Autodesk Fusion 360 part; units mm, degrees
sketch "Sketch1" plane through (0, 0, 0) normal (1, 0, 0) x (0, 1, 0)
  line L0 (15.2, 10) -> (-15.2, 10)
  line L1 (-15.2, 10) -> (-15.2, -10)
  line L2 (-15.2, -10) -> (15.2, -10)
  line L3 (15.2, -10) -> (15.2, 10)
  line L4 (15.2, 10) -> (-15.2, -10) construction
  line L5 (-15.2, 10) -> (15.2, -10) construction
  line L6 (0, 10) -> (0, -10)
  line L7 (15.2, 10) -> (15.2, 8.5)
  line L8 (15.2, 8.5) -> (13.7, 8.5)
  line L9 (13.7, 8.5) -> (13.7, 6.5)
  line L10 (13.7, 6.5) -> (15.2, 6.5)
  line L11 (15.2, -10) -> (15.2, -8.5)
  line L12 (15.2, -8.5) -> (13.7, -8.5)
  line L13 (13.7, -8.5) -> (13.7, -6.5)
  line L14 (13.7, -6.5) -> (15.2, -6.5)
  line L15 (15.2, -6.5) -> (15.2, -5)
  line L16 (15.2, -5) -> (13.2, -5)
  line L17 (15.2, 6.5) -> (15.2, 5)
  line L18 (15.2, 5) -> (13.2, 5)
  line L19 (13.2, 5) -> (13.2, -5)
  dimension "d1" = 30.4
  dimension "d2" = 20
  dimension "d3" = 1.5
  dimension "d4" = 1.5
  dimension "d5" = 2
  dimension "d6" = 1.5
  dimension "d7" = 1.5
  dimension "d8" = 2
  dimension "d9" = 1.5
  dimension "d10" = 2
  dimension "d11" = 2
revolve "Revolve1" add sketch "Sketch1" angle 360 about axis through (0, 0, 10) along (0, 0, -1) contours L0 L2 L3 L6 L7 L8 L9 L10 L11 L12 L13 L14 L15 L16 L17 L18 L19
sketch "Sketch2" plane through (0, 0, 10) normal (0, 0, 1) x (-1, 0, 0)
  circle A0 centre (0, 0) radius 15.2
  line L0 (5.588, -5.588) -> (-5.588, -5.588)
  line L1 (-5.588, -5.588) -> (-5.588, 5.588)
  line L2 (-5.588, 5.588) -> (5.588, 5.588)
  line L3 (5.588, 5.588) -> (5.588, -5.588)
  line L4 (5.588, -5.588) -> (-5.588, 5.588) construction
  line L5 (-5.588, -5.588) -> (5.588, 5.588) construction
  circle A1 centre (5.588, -5.588) radius 1.5875
  dimension "d13" = 11.176
  dimension "d14" = 11.176
  dimension "d15" = 3.175
extrude "Extrude1" cut sketch "Sketch2" against normal blind 25 contours L0 L3 A1 | L0 L3 A1
pattern_circular "C-Pattern1" count 4 over 360 about axis through (0, 0, 1.75) along (0, 0, 1) of "Extrude1"
chamfer "Chamfer1" distance 1.5 angle 45 1 edges at (-12.7729, 4.9541, -8.5)
chamfer "Chamfer2" distance 2 angle 45 1 edges at (-12.3067, 4.7733, -5)
chamfer "Chamfer3" distance 1.5 angle 45 1 edges at (-12.7729, 4.9541, 6.5)
sketch "Sketch3" plane through (0, 0, -10) normal (0, 0, -1) x (1, 0, 0)
  circle A0 centre (5.588, -5.588) radius 1.5875
  circle A1 centre (5.588, 5.588) radius 1.5875
  circle A2 centre (-5.588, 5.588) radius 1.5875
  circle A3 centre (-5.588, -5.588) radius 1.5875
  circle A4 centre (0, 0) radius 15.2
  circle A5 centre (-5.588, 5.588) radius 2.5
  circle A6 centre (-5.588, -5.588) radius 2.5
  circle A7 centre (5.588, -5.588) radius 2.5
  circle A8 centre (5.588, 5.588) radius 2.5
  dimension "d23" = 5
  dimension "d24" = 5
  dimension "d25" = 5
  dimension "d26" = 5
extrude "Extrude2" cut sketch "Sketch3" against normal blind 15 contours A5 | A6 | A7 | A8
sketch "Sketch4" plane through (0, 0, 10) normal (0, 0, 1) x (-1, 0, 0)
  circle A0 centre (-5.588, -5.588) radius 1.5875
  circle A1 centre (-5.588, 5.588) radius 1.5875
  circle A2 centre (5.588, 5.588) radius 1.5875
  circle A3 centre (5.588, -5.588) radius 1.5875
  circle A4 centre (0, 0) radius 15.2
  circle A5 centre (0, 0) radius 4.7625
  dimension "d29" = 9.525
extrude "Extrude3" cut sketch "Sketch4" against normal blind 26 contours A5
equation "d13 = 0.315 in + 0.125 in"
equation "d14 = 0.315 in + 0.125 in"
Verification items for the finished model (mm, model axes). A direction names the side the tool comes from. Give positions to 0.01 mm unless a question says otherwise; leave off trailing zeros. Write each loop counter-clockwise with the first axis right and the second up, starting at its lowest first coordinate (ties: lowest second). Pieces come first, ordered by that corner, then holes.
(1) Mould release check, pull along Y, two halves, no side actions. Record for faces 1 (the face through (3.78, 2.9, 0.14)), 2 (the face through (3.75, -7.28, -2.61)), 3 (the face through (4, 3, 10)), 4 (the face through (-0.668, -15.185, -5.74)): +Y half, -Y half, draft (parallel to the pull), parting line (faces both ways), or undercut.
(2) Gauge pin test, flat ends, axial feed: pin 1 (3 mm diameter, centred on x = 5.588, y = -5.588, fed in from +Z); pin 2 (12 mm diameter, centred on y = 9, z = 3, fed in from +X); pin 3 (6 mm diameter, centred on y = -10.5, z = -5.5, fed in from -X); pin 4 (5 mm diameter, centred on x = 8, z = -4.5, fed in from +Y). Record the tip position at first contact, or that the pin passes through.
(3) Material ranges on line 1 (X direction, y = 7.5, z = 4.5); line 2 (X direction, y = 6.5, z = -1); line 3 (Y direction, x = 3.5, z = 9), recorded low to high.
(4) Access from +Z, -Z, +X, -X, +Y, -Y to the whole of each face (thin tool, end or side, straight path). Record for faces 5 (the face through (4, 4, 5)), 6 (the face through (6.554, 4.328, 7.535)), 7 (the face through (14, -2, 8.5)).
(5) Cross-section at A-A (z = 1.5). Enter the section's corners in (x, y) (1 decimal).
(6) Cross-section at B-B (y = 6). State how many separate pieces and enclosed holes the cut face has, plus the area to 3 significant figures.
Worked out:
1. face 1: undercut
1. face 2: undercut
1. face 3: draft
1. face 4: parting line
2. pin 1: passes through
2. pin 2: stops at x = 14.83
2. pin 3: stops at x = -13.22
2. pin 4: stops at y = 14.15
3. line 1: x = -10.86 to -7.2, -3.98 to 3.98, 7.2 to 10.86
3. line 2: x = -11.49 to -7.92, -3.26 to 3.26, 7.92 to 11.49
3. line 3: y = -14.79 to -3.23, 3.23 to 14.79
4. face 5: -Z
4. face 6: +Z, -Z
4. face 7: none
5. outline: circle Ø26.4 at (0, 0); hole circle Ø5 at (-5.6, -5.6); hole circle Ø5 at (-5.6, 5.6); hole circle Ø9.5 at (0, 0); hole circle Ø5 at (5.6, -5.6); hole circle Ø5 at (5.6, 5.6)
6. separate pieces: 3
6. enclosed holes: 0
6. area: 332 mm2
